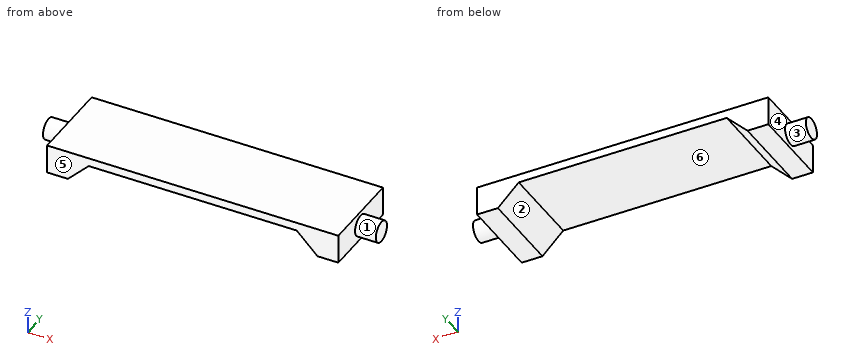
```python
from build123d import *

# Parameters (mm, degrees)
SKETCH1_W           = 700
SKETCH1_H           = 200
BOSS_EXTRUDE1_DEPTH = 70
CUT_EXTRUDE1_DEPTH  = 201
SKETCH3_R           = 25
BOSS_EXTRUDE2_DEPTH = 50
SKETCH4_R           = 25
BOSS_EXTRUDE3_DEPTH = 50


with BuildPart() as part:
    # Sketch1 → Boss-Extrude1 (new body)
    with BuildSketch(Plane.XY):
        Rectangle(SKETCH1_W, SKETCH1_H)
    extrude(amount=BOSS_EXTRUDE1_DEPTH)

    # Sketch2 → Cut-Extrude1 (cut, through all)
    with BuildSketch(Plane.XZ.offset(100)):
        Polygon((-300, 0), (-250, 50), (250, 50), (300, 0), align=None)
    extrude(amount=-CUT_EXTRUDE1_DEPTH, mode=Mode.SUBTRACT)

    # Sketch3 → Boss-Extrude2 (add)
    with BuildSketch(Plane.ZY.offset(350)):
        with Locations((35, 0)):
            Circle(SKETCH3_R)
    extrude(amount=BOSS_EXTRUDE2_DEPTH)

    # Sketch4 → Boss-Extrude3 (add)
    with BuildSketch(Plane(origin=(350, 0, 0), x_dir=(0, 0, -1), z_dir=(1, 0, 0))):
        with Locations((-35, 0)):
            Circle(SKETCH4_R)
    extrude(amount=BOSS_EXTRUDE3_DEPTH)


solid = part.part
```
Read the model definition and answer for the solid it produces. Units are mm, in the model's axes. Face numbers are marked on the shaded views. A direction names the side the tool comes from. Round coordinates to 2 decimals unless told otherwise and drop trailing zeros. Loops run counter-clockwise (first coordinate to the right, second up) from the corner with the lowest first, then second, coordinate; pieces in that order, holes last. Notation, with made-up numbers: (1, 58.5) -> (19, 58.5) arc R14 ccw to (19, 64.5) -> close; hole circle Ø2 at (18, -9.75). An arc over 180 degrees is marked (long way). One line per item, written item: value.
1) For the marked faces 1, 2 and 3, determine the directions among +Z, -Z, +X, -X, +Y, -Y from which every point of the face is accessible in a straight line to the end or side of a thin tool.
Answer list:
face 1: +X
face 2: -Z, +Y, -Y
face 3: -X
2) A cutting plane is placed at B-B (y = 0). Determine the outline of the cut face in (x, z), and give its area (3 significant figures).
Answer list:
outline: (-400, 10) -> (-350, 10) -> (-350, 0) -> (-300, 0) -> (-250, 50) -> (250, 50) -> (300, 0) -> (350, 0) -> (350, 10) -> (400, 10) -> (400, 60) -> (350, 60) -> (350, 70) -> (-350, 70) -> (-350, 60) -> (-400, 60) -> close
area: 26,500 mm²
3) A cutting plane is placed at A-A (z = 35). Determine the outline of the cut face in (x, y).
Answer list:
outline: (-400, -25) -> (-350, -25) -> (-350, -100) -> (-265, -100) -> (-265, 100) -> (-350, 100) -> (-350, 25) -> (-400, 25) -> close; (265, -100) -> (350, -100) -> (350, -25) -> (400, -25) -> (400, 25) -> (350, 25) -> (350, 100) -> (265, 100) -> close
4) Consider L1, parallel to Z at x = 174.5, y = 67.5; L2, parallel to X at y = -31.5, z = 13; L3, parallel to X at y = 63, z = 47. Determine where each line is inside the solid, lowest interval first. Write a range as [from, to].
Answer list:
L1: z = [50, 70]
L2: x = [-350, -287], [287, 350]
L3: x = [-350, -253], [253, 350]
5) The mould has two halves that part along X. Classify the marked faces 4, 5 and 6: pulls with the +X half, pulls with the -X half, needs draft (parallel to the pull), parting line crosses it, or undercut.
Answer list:
face 4: pulls with the -X half
face 5: needs draft
face 6: undercut
6) Flat-ended cylindrical pins translate along their axes: P1, Ø2, axis at y = -53, z = 16, coming from the -X side; P2, Ø8, axis at x = -181, y = 59.5, coming from the -Z side. Find the tip coordinate at first contact, or state that the pin passes through.
Answer list:
P1: stops at x = -350
P2: stops at z = 50
7) A cutting plane is placed at D-D (y = 32.5). Determine the outline of the cut face in (x, z), and give its area (3 significant figures).
Answer list:
outline: (-350, 0) -> (-300, 0) -> (-250, 50) -> (250, 50) -> (300, 0) -> (350, 0) -> (350, 70) -> (-350, 70) -> close
area: 21,500 mm²
8) A cutting plane is placed at C-C (x = 51). Determine the outline of the cut face in (y, z), and give its area (3 significant figures).
Answer list:
outline: (-100, 50) -> (100, 50) -> (100, 70) -> (-100, 70) -> close
area: 4,000 mm²
